Build history of the part. All positions in model axes, mm. Face numbers are marked on the shaded views. Round coordinates to 2 decimals unless told otherwise and drop trailing zeros. Write each loop counter-clockwise with the first axis right and the second up, starting at its lowest first coordinate (ties: lowest second). Pieces come first, ordered by that corner, then holes. Notation, with made-up numbers: M 56.5,14 L 109.5,14 A13 ccw 109.5,31 Z; hole C 30,-30 d2. An arc over 180 degrees is marked long. One line per item, written item: value. Start each with the question number.
```python
from build123d import *

# Parameters (mm, degrees)
F0_R     = 50.8
F0_R_2   = 2.54
F0_R_3   = 31.75
F1_DEPTH = 25.4


with BuildPart() as f1:
    # F0 (on Front) → F1 (new body, symmetric)
    with BuildSketch(Plane.XZ):
        Circle(F0_R)
        with Locations((0, -41.275)):
            Circle(F0_R_2, mode=Mode.SUBTRACT)
        with Locations((-41.275, 0)):
            Circle(F0_R_2, mode=Mode.SUBTRACT)
        Circle(F0_R_3, mode=Mode.SUBTRACT)
        with Locations((41.275, 0)):
            Circle(F0_R_2, mode=Mode.SUBTRACT)
        with Locations((0, 41.275)):
            Circle(F0_R_2, mode=Mode.SUBTRACT)
    extrude(amount=F1_DEPTH, both=True)


solid = f1.part
```
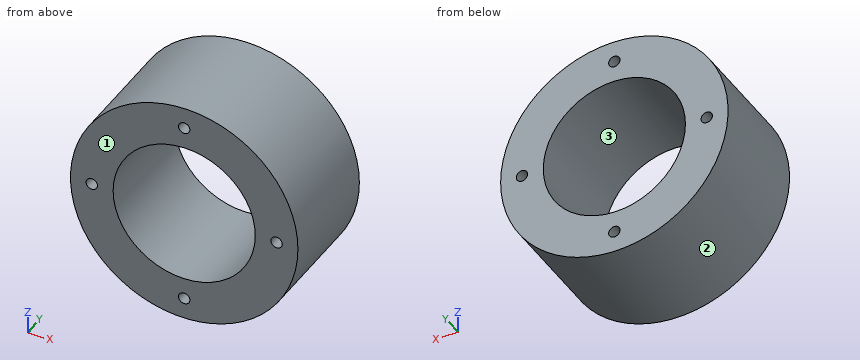
Item 1: Two-plate mould, pull along X, no slides. Class the marked faces 1, 2 and 3: pulls with the +X half, pulls with the -X half, needs draft (parallel to the pull), parting line crosses it, or undercut.
Item 2: Drop flat-ended pins along their axis: pin 1 (6.5 mm diameter, centred on x = 41.275, z = 0, fed in from +Y); pin 2 (6 mm diameter, centred on x = -6.5, y = -18.5, fed in from -Z); pin 3 (8 mm diameter, centred on x = -1.5, y = -13.5, fed in from +Z); pin 4 (12 mm diameter, centred on y = 14, z = -25.5, fed in from +X). Give the stop position or say it passes through.
Item 3: Cut at A-A, the plane z = 0. Write the cut outline in (x, y) (3 decimals), plus the area to 3 significant figures.
Item 4: Drill centre lines: line 1 (Z direction, x = 0, y = 10) (3 decimals); line 2 (Z direction, x = 1.5, y = -14); line 3 (X direction, y = -4.5, z = -22.5). Where is each one in solid material? Low to high.
Item 5: Cut at B-B, the plane x = 0. Write the cut outline in (y, z) (3 decimals).
Item 6: Cut at C-C, the plane y = -19. Write the cut outline in (x, z) (3 decimals), plus the area to 3 significant figures.
Item 7: Cut at D-D, the plane x = 33.5. Write the cut outline in (y, z).
Computed values:
1. face 1: needs draft
1. face 2: parting line crosses it
1. face 3: undercut
2. pin 1: stops at y = 25.4
2. pin 2: stops at z = -50.68
2. pin 3: stops at z = 50.8
2. pin 4: stops at x = 46.91
3. outline: M -50.8,-25.4 L -43.815,-25.4 L -43.815,25.4 L -50.8,25.4 Z; M -38.735,-25.4 L -31.75,-25.4 L -31.75,25.4 L -38.735,25.4 Z; M 31.75,-25.4 L 38.735,-25.4 L 38.735,25.4 L 31.75,25.4 Z; M 43.815,-25.4 L 50.8,-25.4 L 50.8,25.4 L 43.815,25.4 Z
3. area: 1,420 mm2
4. line 1: z = -50.8 to -43.815, -38.735 to -31.75, 31.75 to 38.735, 43.815 to 50.8
4. line 2: z = -50.78 to -43.32, -39.23 to -31.71, 31.71 to 39.23, 43.32 to 50.78
4. line 3: x = -45.55 to -22.4, 22.4 to 45.55
5. outline: M -25.4,-50.8 L 25.4,-50.8 L 25.4,-43.815 L -25.4,-43.815 Z; M -25.4,-38.735 L 25.4,-38.735 L 25.4,-31.75 L -25.4,-31.75 Z; M -25.4,31.75 L 25.4,31.75 L 25.4,38.735 L -25.4,38.735 Z; M -25.4,43.815 L 25.4,43.815 L 25.4,50.8 L -25.4,50.8 Z
6. outline: C 0,0 d101.6; hole C -41.275,0 d5.08; hole C 0,0 d63.5; hole C 0,-41.275 d5.08; hole C 0,41.275 d5.08; hole C 41.275,0 d5.08
6. area: 4,860 mm2
7. outline: M -25.4,-38.19 L 25.4,-38.19 L 25.4,38.19 L -25.4,38.19 Z
